```python
from build123d import *

# Parameters (mm, degrees)
F0_W     = 13.5
F0_H     = 24.5
F0_W_2   = 11.5
F0_H_2   = 22.5
F1_DEPTH = 13
F2_W     = 13.5
F2_H     = 24.5
F2_W_2   = 11.5
F2_H_2   = 22.5
F3_DEPTH = 3


with BuildPart() as f1:
    # F0 (on Front) → F1 (new body)
    with BuildSketch(Plane.XZ):
        Rectangle(F0_W, F0_H)
        Rectangle(F0_W_2, F0_H_2, mode=Mode.SUBTRACT)
    extrude(amount=F1_DEPTH)

    # F2 (on face) → F3 (join)
    with BuildSketch(Plane.XZ.offset(13)):
        Polygon((-20, 51.75), (-20, -12.25), (-6.75, -12.25), (-6.75, 12.25), (6.75, 12.25), (6.75, -12.25), (20, -12.25), (20, 51.75), align=None)
        Rectangle(F2_W, F2_H)
        Rectangle(F2_W_2, F2_H_2, mode=Mode.SUBTRACT)
        Rectangle(F2_W_2, F2_H_2)
    extrude(amount=F3_DEPTH)


solid = f1.part
```
Check sheet for the modelled part. Datum: model origin and axes. Units: mm. A direction names the side the tool comes from. Coordinates: 2 decimals unless noted, no trailing zeros. Write each loop counter-clockwise with the first axis right and the second up, starting at its lowest first coordinate (ties: lowest second). Pieces come first, ordered by that corner, then holes. Notation, with made-up numbers: (-9, 64) -> (23, 64) arc R13 cw to (23, 87) -> close; hole circle Ø9 at (67.25, 61.5). An arc over 180 degrees is marked (long way). Use a Markdown table: item, result.
1. Sectioned sample at C-C (x = -0.5). Enter the section's corners in (y, z), plus the area to 3 significant figures.
Reported:
| item | result |
|---|---|
| outline | (-16, -12.25) -> (0, -12.25) -> (0, -11.25) -> (-13, -11.25) -> (-13, 11.25) -> (0, 11.25) -> (0, 12.25) -> (-13, 12.25) -> (-13, 51.75) -> (-16, 51.75) -> close |
| area | 218 mm2 |
2. Release check for a two-part mould opening along Z. For faces 5 (the flat face through (0, -6, 12.25)), 6 (the flat face through (0, -16, 20)), 7 (the flat face through (5.75, -6, 0)) record: pulls with the +Z half, pulls with the -Z half, needs draft (parallel to the pull), parting line crosses it, or undercut.
Reported:
| item | result |
|---|---|
| face 5 | pulls with the +Z half |
| face 6 | needs draft |
| face 7 | undercut |
3. Tool access check on faces 1 (the flat face through (0, -6, -11.25)), 2 (the flat face through (-6.75, -6, 0)), 3 (the flat face through (6.75, -6, 0)), 4 (the flat face through (0, -14, 51.75)). Record the directions out of +Z, -Z, +X, -X, +Y, -Y that give a thin tool (end or side, any length) a straight path to the whole face; none if there is none.
Reported:
| item | result |
|---|---|
| face 1 | +Y |
| face 2 | +Z, -Z, -X, +Y |
| face 3 | +Z, -Z, +X, +Y |
| face 4 | +Z, +X, -X, +Y, -Y |
4. Go/stop test with flat-tipped pins: pin 1 Ø12.5 at (x, z) = (1, -3.5) entering from +Y; pin 2 Ø6.5 at (y, z) = (-7.5, -3.5) entering from +X; pin 3 Ø5 at (x, z) = (13.5, -4.5) entering from +Y; pin 4 Ø6 at (x, y) = (-2.5, -7) entering from +Z. Record where each tip stops, or that it passes through.
Reported:
| item | result |
|---|---|
| pin 1 | stops at y = 0 |
| pin 2 | stops at x = 6.75 |
| pin 3 | stops at y = -13 |
| pin 4 | stops at z = 12.25 |
5. Sectioned sample at B-B (y = -9.75). Enter the section's corners in (x, z).
Reported:
| item | result |
|---|---|
| outline | (-6.75, -12.25) -> (6.75, -12.25) -> (6.75, 12.25) -> (-6.75, 12.25) -> close; hole (-5.75, -11.25) -> (5.75, -11.25) -> (5.75, 11.25) -> (-5.75, 11.25) -> close |
6. Scan lines: line 1 along Z through (x, y) = (-5, -12.5); line 2 along X through (y, z) = (-7.25, 8); line 3 along Y through (x, z) = (15, 32). Record each from-to range of solid material in increasing order.
Reported:
| item | result |
|---|---|
| line 1 | z = -12.25 to -11.25, 11.25 to 12.25 |
| line 2 | x = -6.75 to -5.75, 5.75 to 6.75 |
| line 3 | y = -16 to -13 |
7. Sectioned sample at A-A (z = 7). Enter the section's corners in (x, y), plus the area to 3 significant figures.
Reported:
| item | result |
|---|---|
| outline | (-20, -16) -> (20, -16) -> (20, -13) -> (6.75, -13) -> (6.75, 0) -> (5.75, 0) -> (5.75, -13) -> (-5.75, -13) -> (-5.75, 0) -> (-6.75, 0) -> (-6.75, -13) -> (-20, -13) -> close |
| area | 146 mm2 |
8. Sectioned sample at D-D (z = 28). Enter the section's corners in (x, y), plus the area to 3 significant figures.
Reported:
| item | result |
|---|---|
| outline | (-20, -16) -> (20, -16) -> (20, -13) -> (-20, -13) -> close |
| area | 120 mm2 |
